Here's how the part is built. I have some questions about the finished solid (model axes, mm). Give positions to 0.01 mm unless a question says otherwise; leave off trailing zeros. Order: outer loops, then holes, each group sorted by start corner. A loop starts at its lowest first (then second) coordinate and runs counter-clockwise, first axis right, second up.
Autodesk Inventor part; units mm, degrees
ref_plane "YZ Plane" through (0, 0, 0) normal (1, 0, 0) x (0, 1, 0)
ref_plane "XZ Plane" through (0, 0, 0) normal (0, 1, 0) x (-1, 0, 0)
ref_plane "XY Plane" through (0, 0, 0) normal (0, 0, 1) x (1, 0, 0)
sketch "Sketch1" plane through (0, 0, 0) normal (0, 0, 1) x (1, 0, 0)
  arc A0 (-3.175, 3.175) -> (0, 0) centre (0.0002, 3.1752) ccw
  line L0 (44.45, 0) -> (0, 0)
  arc A1 (44.45, 0) -> (47.625, 3.175) centre (44.4498, 3.1752) ccw
  line L1 (47.625, 79.375) -> (47.625, 3.175)
  arc A2 (47.625, 79.375) -> (44.45, 82.55) centre (44.4498, 79.3748) ccw
  line L2 (0, 82.55) -> (44.45, 82.55)
  arc A3 (0, 82.55) -> (-3.175, 79.375) centre (0.0002, 79.3748) ccw
  line L3 (-3.175, 3.175) -> (-3.175, 79.375)
  circle A4 centre (0, 3.175) radius 1.6
  circle A5 centre (7.112, 4.191) radius 0.51
  circle A6 centre (7.112, 9.271) radius 0.51
  circle A7 centre (7.112, 6.731) radius 0.51
  circle A8 centre (9.652, 6.731) radius 0.51
  circle A9 centre (9.652, 4.191) radius 0.51
  circle A10 centre (9.652, 9.271) radius 0.51
  circle A11 centre (15.655, 10.499) radius 1.15
  circle A12 centre (14.225, 36.449) radius 0.85
  circle A13 centre (4.699, 60.198) radius 0.51
  circle A14 centre (4.699, 57.658) radius 0.51
  circle A15 centre (0, 79.375) radius 1.6
  circle A16 centre (4.699, 62.738) radius 0.51
  circle A17 centre (4.699, 65.278) radius 0.51
  circle A18 centre (13.7, 69.341) radius 0.46
  circle A19 centre (16.2, 69.341) radius 0.46
  circle A20 centre (6.13, 72.051) radius 1.15
  circle A21 centre (11.7, 69.341) radius 0.46
  circle A22 centre (9.2, 69.341) radius 0.46
  circle A23 centre (23.225, 13.209) radius 0.46
  circle A24 centre (25.725, 13.209) radius 0.46
  circle A25 centre (18.725, 13.209) radius 0.46
  circle A26 centre (21.225, 13.209) radius 0.46
  circle A27 centre (28.795, 10.499) radius 1.15
  circle A28 centre (44.45, 3.175) radius 1.6
  circle A29 centre (30.225, 36.449) radius 0.85
  circle A30 centre (39.751, 57.531) radius 0.51
  circle A31 centre (39.751, 60.071) radius 0.51
  circle A32 centre (31.385, 69.341) radius 0.46
  circle A33 centre (33.385, 69.341) radius 0.46
  circle A34 centre (19.27, 72.051) radius 1.15
  circle A35 centre (28.885, 69.341) radius 0.46
  circle A36 centre (25.815, 72.051) radius 1.15
  circle A37 centre (39.751, 65.151) radius 0.51
  circle A38 centre (39.751, 62.611) radius 0.51
  circle A39 centre (35.885, 69.341) radius 0.46
  circle A40 centre (38.955, 72.051) radius 1.15
  circle A41 centre (44.45, 79.375) radius 1.6
  line L4 (19.2278, 19.1042) -> (19.2278, 22.8146) construction
  line L5 (20.234, 18.0978) -> (19.2662, 19.0663) construction
  line L6 (20.2568, 18.0747) -> (24.1988, 18.0747) construction
  line L7 (19.2662, 22.8525) -> (20.234, 23.821) construction
  line L8 (24.1988, 23.8441) -> (20.2568, 23.8441) construction
  line L9 (24.2216, 23.821) -> (25.1894, 22.8525) construction
  line L10 (25.2278, 22.8146) -> (25.2278, 19.1042) construction
  line L11 (25.1894, 19.0663) -> (24.2216, 18.0978) construction
  line L12 (19.2278, 23.8441) -> (25.2278, 23.8441) construction
  line L13 (25.2278, 23.8441) -> (25.2278, 18.0747) construction
  line L14 (25.2278, 18.0747) -> (19.2278, 18.0747) construction
  line L15 (19.2278, 18.0747) -> (19.2278, 23.8441) construction
  line L16 (19.2278, 20.9594) -> (25.2278, 20.9594) construction
  line L17 (22.2278, 23.8441) -> (22.2278, 18.0747) construction
  line L18 (15.8778, 27.3094) -> (28.5778, 27.3094)
  line L19 (28.5778, 27.3094) -> (28.5778, 14.6094)
  line L20 (28.5778, 14.6094) -> (15.8778, 14.6094)
  line L21 (15.8778, 14.6094) -> (15.8778, 27.3094)
  line L22 (15.8778, 27.3094) -> (28.5778, 14.6094) construction
  line L23 (28.5778, 27.3094) -> (15.8778, 14.6094) construction
  point P0 (22.2278, 20.9594)
  dimension "d0" = 12.7
  dimension "d1" = 12.7
extrude "Extrusion1" add sketch "Sketch1" along normal blind 3 contours L3 A3 L2 A2 L1 A1 L0 A0 | A5 | A6 | A7 | A8 | A9 | A10 | A11 | A12 | A13 | A14 | A16 | A17 | A18 | A19 | A20 | A21 | A22 | A23 | A24 | A25 | A26 | A27 | A29 | A30 | A31 | A32 | A33 | A34 | A35 | A36 | A37 | A38 | A39 | A40
fillet "Fillet1" radius 3 4 edges at (15.8778, 27.3094, 1.5) (28.5778, 27.3094, 1.5) (15.8778, 14.6094, 1.5) (28.5778, 14.6094, 1.5)
sketch "Sketch2" plane through (0, 0, 3) normal (0, 0, 1) x (1, 0, 0)
  line L0 (-3.175, 79.375) -> (-3.175, 3.175) construction
  arc A0 (-3.175, 3.175) -> (0, 0) centre (0.0002, 3.1752) ccw construction
  line L1 (0, 0) -> (44.45, 0) construction
  arc A1 (44.45, 0) -> (47.625, 3.175) centre (44.4498, 3.1752) ccw construction
  line L2 (47.625, 3.175) -> (47.625, 79.375) construction
  arc A2 (47.625, 79.375) -> (44.45, 82.55) centre (44.4498, 79.3748) ccw construction
  line L3 (44.45, 82.55) -> (0, 82.55) construction
  arc A3 (0, 82.55) -> (-3.175, 79.375) centre (0.0002, 79.3748) ccw construction
  line L4 (18.8778, 27.3094) -> (25.5778, 27.3094) construction
  arc A4 (28.5778, 24.3094) -> (25.5778, 27.3094) centre (25.5778, 24.3094) ccw construction
  line L5 (28.5778, 24.3094) -> (28.5778, 17.6094) construction
  arc A5 (25.5778, 14.6094) -> (28.5778, 17.6094) centre (25.5778, 17.6094) ccw construction
  line L6 (25.5778, 14.6094) -> (18.8778, 14.6094) construction
  arc A6 (15.8778, 17.6094) -> (18.8778, 14.6094) centre (18.8778, 17.6094) ccw construction
  line L7 (15.8778, 17.6094) -> (15.8778, 24.3094) construction
  arc A7 (18.8778, 27.3094) -> (15.8778, 24.3094) centre (18.8778, 24.3094) ccw construction
  circle A8 centre (44.45, 79.375) radius 1.6 construction
  circle A9 centre (44.45, 3.175) radius 1.6 construction
  circle A10 centre (0, 79.375) radius 1.6 construction
  circle A11 centre (0, 3.175) radius 1.6 construction
  circle A12 centre (22.225, 53.467) radius 12.4968
  line L8 (22.225, 82.55) -> (22.225, 0) construction
  line L9 (0, 0) -> (44.45, 0) construction
  line L10 (18.1055, 65.2653) -> (26.3445, 65.2653)
  line L11 (18.1055, 41.6687) -> (26.3445, 41.6687)
  line L12 (22.225, 65.9638) -> (22.225, 65.2653) construction
  line L13 (22.225, 41.6687) -> (22.225, 40.9702) construction
  dimension "d5" = 24.9936
  dimension "d6" = 53.467
  dimension "d7" = 23.5966
  dimension "d8" = 0.6985
  dimension "d9" = 0.6985
extrude "Extrusion2" cut sketch "Sketch2" against normal through all contours A12 L11 L10
equation "\"d1\" = d0"
equation "\"d9\" = d8"
properties part number "Cover"
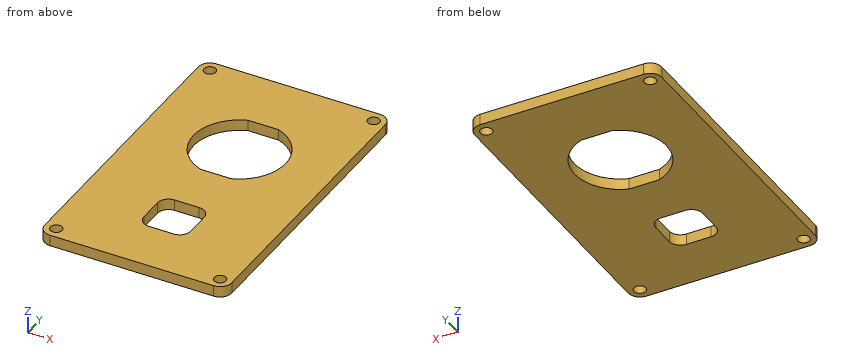
Q1. I need wall thicknesses on L1, parallel to Y at x = 24, z = 0.8; L2, parallel to Y at x = 0, z = 1.25 (3 decimals); L3, parallel to X at y = 24.5, z = 1.5 (3 decimals). Which ranges of each line are inside material? Lowest first, please.
Filled sheet:
L1: y = 0 to 14.61, 27.31 to 41.67, 65.27 to 82.55
L2: y = 0 to 1.575, 4.775 to 77.775, 80.975 to 82.55
L3: x = -3.175 to 15.884, 28.572 to 47.625
Q2. If we section it at B-B on z = 1.45: Give the number of separate pieces and of enclosed holes in the cut face, plus the area to 3 significant figures.
Filled sheet:
separate pieces: 1
enclosed holes: 6
area: 3,520 mm2
Q3. I'm going to push a flat-ended pin straight in: P1, Ø3, axis at x = 0, y = 3.175, coming from the +Z side. Where does the tip first touch, or does it pass through?
Filled sheet:
P1: passes through
Q4. If we section it at C-C on x = 32.5: List the corners of the cut face in (y, z) for me, plus the area to 3 significant figures.
Filled sheet:
outline: (0, 0) - (46.35, 0) - (46.35, 3) - (0, 3) - close; (60.58, 0) - (82.55, 0) - (82.55, 3) - (60.58, 3) - close
area: 205 mm2
Q5. If we section it at A-A on y = 50: List the corners of the cut face in (x, z) for me (3 decimals), plus the area to 3 significant figures.
Filled sheet:
outline: (-3.175, 0) - (10.219, 0) - (10.219, 3) - (-3.175, 3) - close; (34.231, 0) - (47.625, 0) - (47.625, 3) - (34.231, 3) - close
area: 80.4 mm2
